Check sheet for the modelled part. Datum: model origin and axes. Units: mm. A direction names the side the tool comes from. Coordinates: 2 decimals unless noted, no trailing zeros. Order: outer loops, then holes, each group sorted by start corner. A loop starts at its lowest first (then second) coordinate and runs counter-clockwise, first axis right, second up.
Autodesk Inventor part; units mm, degrees
ref_plane "YZ Plane" through (0, 0, 0) normal (1, 0, 0) x (0, 1, 0)
ref_plane "XZ Plane" through (0, 0, 0) normal (0, 1, 0) x (-1, 0, 0)
ref_plane "XY Plane" through (0, 0, 0) normal (0, 0, 1) x (1, 0, 0)
sketch "Skizze10" plane through (0, 0, 0) normal (1, 0, 0) x (0, 1, 0)
  arc A0 (0, -9.6) -> (0, 9.6) centre (0, 0) ccw
  line L0 (0, 0) -> (0, -20)
  line L1 (0, 0) -> (0, 24.5)
  line L2 (-2.8, 0) -> (16.8, 0)
  line L3 (0, 24.5) -> (9.5, 24.5)
  line L4 (9.5, 24.5) -> (9.5, 10.2835)
  arc A1 (9.5, -10.2835) -> (9.5, 10.2835) centre (0, 0) ccw
  line L5 (9.5, -10.2835) -> (9.5, -20)
  line L6 (0, -20) -> (9.5, -20)
  point P0 (0, 9.6)
  dimension "d79" = 9.6
  dimension "d80" = 20
  dimension "d81" = 24.5
  dimension "d84" = 9.5
  dimension "d85" = 14
extrude "Extrusion9" add sketch "Skizze10" along normal mid plane 8.5 contours A0 L2 A1 L5 L6 L0 | A0 L1 L3 L4 A1 L2
sketch "Skizze11" plane through (0, 0, 0) normal (0, 1, 0) x (-1, 0, 0)
  circle A0 centre (0, -13.45) radius 1.7
  circle A1 centre (0, 13.45) radius 1.7
  line L0 (-4.25, -20) -> (-4.25, -10.2835)
  line L1 (0, -27.03) -> (0, 22.18)
  point P0 (0, 0)
  dimension "d88" = 13.45
  dimension "d89" = 13.45
  dimension "d90" = 3.4
  dimension "d91" = 3.4
extrude "Extrusion10" cut sketch "Skizze11" along normal through all
sketch "Skizze12" plane through (0, 0, 0) normal (0, 1, 0) x (-1, 0, 0)
  line L0 (1.05, 23) -> (-4.25, 23)
  line L1 (-4.25, 18.6) -> (1.05, 18.6)
  line L2 (2.11, 0) -> (-5.31, 0)
  line L3 (-4.25, 10.2835) -> (-4.25, 24.5)
  line L4 (1.05, 23) -> (1.05, 18.6)
  point P0 (0, 0)
  dimension "d94" = 4.4
  dimension "d95" = 5.3
  dimension "d99" = 18.6
extrude "Extrusion11" cut sketch "Skizze12" along normal blind 3.35
properties part number "Lagerhalter2"
(1) Cross-section at C-C (y = 9). Enter the section's corners in (x, z).
Filled in:
outline: (-4.25, -20) - (4.25, -20) - (4.25, -3.34) - (-4.25, -3.34) - close; (-4.25, 3.34) - (4.25, 3.34) - (4.25, 24.5) - (-4.25, 24.5) - close; hole circle Ø3.4 at (0, -13.45); hole circle Ø3.4 at (0, 13.45)
(2) Cross-section at B-B (z = -13.45). Enter the section's corners in (x, y).
Filled in:
outline: (-4.25, 0) - (-1.7, 0) - (-1.7, 9.5) - (-4.25, 9.5) - close; (1.7, 0) - (4.25, 0) - (4.25, 9.5) - (1.7, 9.5) - close
(3) Tool access check on faces 1 (the flat face through (2, 2, 18.6)), 2 (the flat face through (0, 9.5, -16)), 3 (the flat face through (0, 9.5, 17)), 4 (the flat face through (0, 0, -16)). Record the directions out of +Z, -Z, +X, -X, +Y, -Y that give a thin tool (end or side, any length) a straight path to the whole face; none if there is none.
Filled in:
face 1: +X, -Y
face 2: -Z, +X, -X, +Y
face 3: +Z, +X, -X, +Y
face 4: +Z, -Z, +X, -X, -Y
(4) Cross-section at A-A (x = 0). Enter the section's corners in (y, z).
Filled in:
outline: (0, -20) - (9.5, -20) - (9.5, -15.15) - (0, -15.15) - close; (0, -11.75) - (9.5, -11.75) - (9.5, -10.28) arc R14 ccw to (9.5, 10.28) - (9.5, 11.75) - (0, 11.75) - (0, 9.6) arc R9.6 cw to (0, -9.6) - close; (0, 15.15) - (9.5, 15.15) - (9.5, 24.5) - (0, 24.5) - (0, 23) - (3.35, 23) - (3.35, 18.6) - (0, 18.6) - close
(5) Go/stop test with flat-tipped pins: P1, Ø2, axis at x = 2, z = 20.5, coming from the -Y side; P2, Ø1, axis at x = 2.5, z = 17.5, coming from the -Y side; P3, Ø1.5, axis at x = 1.5, y = 11.5, coming from the +Z side; P4, Ø4, axis at x = -1, z = 15, coming from the +Y side. Record where each tip stops, or that it passes through.
Filled in:
P1: stops at y = 3.35
P2: stops at y = 0
P3: stops at z = 8.97
P4: stops at y = 9.5
(6) Cross-section at D-D (z = 19.5). Enter the section's corners in (x, y), and give its area (3 significant figures).
Filled in:
outline: (-4.25, 0) - (-1.05, 0) - (-1.05, 3.35) - (4.25, 3.35) - (4.25, 9.5) - (-4.25, 9.5) - close
area: 63.0 mm2
(7) Thickness scan on probe 1 along X at (y, z) = (3.5, 13.45); probe 2 along Z at (x, y) = (3, 1); probe 3 along Z at (x, y) = (-1.25, 5.5). Record the ranges inside material, lowest first.
Filled in:
probe 1: x = -4.25 to -1.7, 1.7 to 4.25
probe 2: z = -20 to -9.55, 9.55 to 18.6, 23 to 24.5
probe 3: z = -20 to -14.6, -12.3 to -7.87, 7.87 to 12.3, 14.6 to 24.5
(8) Release check for a two-part mould opening along X. For faces 5 (the cylindrical face through (0.37, 4.68, 15.11)), 6 (the flat face through (-1.05, 2, 21)), 7 (the cylindrical face through (-0.059, 9.598, 0.211)) record: +X half, -X half, draft (parallel to the pull), parting line (faces both ways), or undercut.
Filled in:
face 5: undercut
face 6: +X half
face 7: draft
